Here's how the part is built. I have some questions about the finished solid (model axes, mm). A direction names the side the tool comes from. Round coordinates to 2 decimals unless told otherwise and drop trailing zeros. Write each loop counter-clockwise with the first axis right and the second up, starting at its lowest first coordinate (ties: lowest second). Pieces come first, ordered by that corner, then holes. Notation, with made-up numbers: (-6.5, 60) -> (-0.5, 60) arc R6 cw to (-0.5, 65) -> close; hole circle Ø8 at (78, 1). An arc over 180 degrees is marked (long way). Answer as CSV lines item,"result".
Autodesk Inventor part; units mm, degrees
ref_plane "YZ Plane" through (0, 0, 0) normal (1, 0, 0) x (0, 1, 0)
ref_plane "XZ Plane" through (0, 0, 0) normal (0, 1, 0) x (-1, 0, 0)
ref_plane "XY Plane" through (0, 0, 0) normal (0, 0, 1) x (1, 0, 0)
sketch "Sketch1" plane through (0, 0, 0) normal (0, 0, 1) x (1, 0, 0)
  line L0 (0, 0) -> (889, 0)
  line L1 (889, 0) -> (889, 50.8)
  line L2 (889, 50.8) -> (0, 50.8)
  line L3 (0, 50.8) -> (0, 0)
  dimension "d0" = 889
  dimension "d1" = 50.8
extrude "Extrusion1" add sketch "Sketch1" along normal blind 25.4
sketch "Sketch2" plane through (0, 0, 25.4) normal (0, 0, 1) x (1, 0, 0)
  line L0 (0, 0) -> (889, 0)
  line L1 (889, 0) -> (889, 12.7)
  line L2 (889, 12.7) -> (0, 12.7)
  line L3 (0, 12.7) -> (0, 0)
  dimension "d4" = 889
  dimension "d5" = 12.7
extrude "Extrusion2" cut sketch "Sketch2" against normal blind 19.05
sketch "Sketch3" plane through (0, 0, 25.4) normal (0, 0, 1) x (1, 0, 0)
  line L0 (0, 50.8) -> (0, 0)
  line L1 (0, 50.8) -> (38.1, 50.8)
  line L2 (38.1, 50.8) -> (38.1, 12.7)
  line L3 (38.1, 12.7) -> (0, 12.7)
  line L4 (0, 12.7) -> (0, 50.8)
  dimension "d8" = 38.1
  dimension "d9" = 38.1
extrude "Extrusion3" cut sketch "Sketch3" against normal blind 12.7
sketch "Sketch4" plane through (0, 0, 25.4) normal (0, 0, 1) x (1, 0, 0)
  line L0 (889, 50.8) -> (850.9, 50.8)
  line L1 (850.9, 50.8) -> (850.9, 12.7)
  line L2 (850.9, 12.7) -> (889, 12.7)
  line L3 (889, 12.7) -> (889, 50.8)
  point P0 (0, 0)
  dimension "d12" = 38.1
  dimension "d13" = 38.1
extrude "Extrusion4" cut sketch "Sketch4" against normal blind 12.7
sketch "Sketch5" plane through (0, 50.8, 0) normal (0, 1, 0) x (1, 0, 0)
  line L0 (0, -6.35) -> (0, -12.7)
  line L1 (0, -12.7) -> (0, -15.875)
  line L2 (0, -15.875) -> (889, -15.875)
  line L3 (889, -15.875) -> (889, -9.525)
  line L4 (889, -12.7) -> (889, -6.35)
  line L5 (889, -9.525) -> (0, -9.525)
  line L6 (0, -9.525) -> (0, -12.7)
  dimension "d22" = 3.175
  dimension "d23" = 889
  dimension "d24" = 889
extrude "Extrusion5" cut sketch "Sketch5" against normal blind 6.35
properties part number "bottomv2" material "Wood (Cherry)"
1. If I drill on line 1 (Z direction, x = 505, y = 49.5) (3 decimals); line 2 (X direction, y = 47, z = 16.25); line 3 (Y direction, x = 76.5, z = 21.5), over which ranges is the centre line in solid material (lowest first)?
Numbers:
line 1,"z = 0 to 9.525, 15.875 to 25.4"
line 2,"x = 38.1 to 850.9"
line 3,"y = 12.7 to 50.8"
2. For pin 1 Ø16 at (x, y) = (876, 33.5) entering from +Z; pin 2 Ø3 at (y, z) = (23, 14.5) entering from -X; pin 3 Ø2 at (x, z) = (469.5, 12) entering from +Y, each with a flat end and sliding along its axis, tell me the tip position at first contact or that it passes through.
Numbers:
pin 1,"stops at z = 12.7"
pin 2,"stops at x = 38.1"
pin 3,"stops at y = 44.45"
3. Suppose I cut it at B-B on y = 29. Please give me the cut outline in (x, z).
Numbers:
outline,"(0, 0) -> (889, 0) -> (889, 12.7) -> (850.9, 12.7) -> (850.9, 25.4) -> (38.1, 25.4) -> (38.1, 12.7) -> (0, 12.7) -> close"
4. Suppose I cut it at A-A on x = 307. Please give me the cut outline in (y, z) (3 decimals).
Numbers:
outline,"(0, 0) -> (50.8, 0) -> (50.8, 9.525) -> (44.45, 9.525) -> (44.45, 15.875) -> (50.8, 15.875) -> (50.8, 25.4) -> (12.7, 25.4) -> (12.7, 6.35) -> (0, 6.35) -> close"
5. On a 3-axis mill with a long thin cutter (end or side, diameter ignored), from which of +Z, -Z, +X, -X, +Y, -Y can I reach the whole of each face in a straight line? I mean faces 1 (the face through (870, 29, 12.7)), 2 (the face through (451, 12.7, 16)), 3 (the face through (438, 26, 0)), 4 (the face through (19, 29, 12.7)), 5 (the face through (439, 32, 25.4)). Say none if no direction works.
Numbers:
face 1,"+Z, +X, +Y, -Y"
face 2,"+Z, +X, -X, -Y"
face 3,"-Z, +X, -X, +Y, -Y"
face 4,"+Z, -X, +Y, -Y"
face 5,"+Z, +X, -X, +Y, -Y"
6. Suppose I cut it at C-C on z = 20. Please give me the cut outline in (x, y), and give its area (3 significant figures).
Numbers:
outline,"(38.1, 12.7) -> (850.9, 12.7) -> (850.9, 50.8) -> (38.1, 50.8) -> close"
area,"31,000 mm^2"
